Autodesk Inventor part; units mm, degrees
ref_plane "YZ Plane" through (0, 0, 0) normal (1, 0, 0) x (0, 1, 0)
ref_plane "XZ Plane" through (0, 0, 0) normal (0, 1, 0) x (-1, 0, 0)
ref_plane "XY Plane" through (0, 0, 0) normal (0, 0, 1) x (1, 0, 0)
sketch "Sketch1" plane through (0, 0, 0) normal (0, 1, 0) x (-1, 0, 0)
  line L0 (3.05, -5.3255) -> (-3.05, -5.3255)
  line L1 (-3.05, -5.3255) -> (-3.05, 4.8245)
  line L2 (-3.05, 4.8245) -> (3.05, 4.8245)
  line L3 (3.05, 4.8245) -> (3.05, -5.3255)
  line L4 (0.9, 4.8245) -> (-0.9, 4.8245)
  line L5 (0.9, 4.8245) -> (0.9, -5.3255)
  line L6 (-0.9, 4.8245) -> (-0.9, -5.3255)
  circle A0 centre (0, 3.486) radius 0.8
  circle A1 centre (-0.0087, -3.8255) radius 0.8
  line L7 (0, 4.8245) -> (0, -5.3255)
  line L8 (-3.05, 0) -> (3.05, 0)
  point P0 (0, 0)
  dimension "d13" = 6.1
  dimension "d44" = 1.8
  dimension "d45" = 2.15
  dimension "d46" = 1.6
  dimension "d47" = 1.6
extrude "Extrusion1" add sketch "Sketch1" along normal blind 10.15 contours L0 L5 L8 L3 | L0 L7 A1 L8 L5 | L8 L5 L2 L3 | L0 L6 L8 L7 A1 | L8 L7 A0 L2 L5 | L0 L1 L8 L6 | L8 L6 L2 L7 A0 | L8 L1 L2 L6
sketch "Sketch11" plane through (-3.05, 0, 4.8245) normal (0, 0, 1) x (1, 0, 0)
  point P0 (3.05, 0)
extrude "Extrusion6" add sketch "Sketch1" against normal blind 1 contours L0 L7 A1 L8 L5 | L0 L6 L8 L7 A1 | L8 L7 A0 L2 L5 | L8 L6 L2 L7 A0
sketch "Sketch12" plane through (0, 10.15, 0) normal (0, 1, 0) x (1, 0, 0)
  circle A0 centre (0.0087, 3.8255) radius 1.265
  circle A1 centre (0, -3.486) radius 1.265
  circle A2 centre (0, -3.486) radius 0.8
  circle A3 centre (0.0087, 3.8255) radius 0.8
  point P0 (0, 0)
  dimension "d52" = 2.53
  dimension "d53" = 2.53
extrude "Extrusion7" cut sketch "Sketch12" against normal blind 1 contours A0 | A1 | A2 | A3
sketch "Sketch13" plane through (-3.05, 10.15, 4.8245) normal (0, 0, 1) x (1, 0, 0)
  line L0 (0, 0) -> (0, -4.15)
  line L1 (0, -10.15) -> (0, 0)
  line L2 (0, -4.15) -> (6.1, -4.15)
  line L3 (6.1, -10.15) -> (6.1, 0)
  line L4 (6.1, 0) -> (6.1, -4.15)
  line L5 (0, 0) -> (6.1, 0)
  point P0 (3.05, -10.15)
  dimension "d56" = 4.15
extrude "Extrusion8" add sketch "Sketch13" along normal blind 17
sketch "Sketch17" plane through (-3.05, 10.15, 21.8245) normal (0, 0, 1) x (1, 0, 0)
  line L0 (6.1, 0) -> (0, 0)
  line L1 (6.1, 0) -> (14.3904, 5.5919)
  line L2 (6.1, 0) -> (16.1, 0) construction
  line L3 (14.3904, 5.5919) -> (10.1964, 11.8097)
  line L4 (10.1964, 11.8097) -> (13.5955, 14.1024)
  line L5 (13.5955, 14.1024) -> (17.7894, 7.8846)
  line L6 (17.7894, 7.8846) -> (19.7132, 5.0325)
  line L7 (6.1, -10.15) -> (6.1, -4.15)
  line L8 (19.7132, 5.0325) -> (6.1, -4.15)
  line L9 (6.1, 0) -> (6.1, -4.15)
  point P0 (3.05, -10.15)
  dimension "d72" = 10
  dimension "d73" = 34
  dimension "d74" = 7.5
  dimension "d75" = 4.1
extrude "Extrusion12" [suppressed]
sketch "Sketch14" plane through (0, 10.15, 0) normal (0, 1, 0) x (1, 0, 0)
  line L0 (3.05, 5.3255) -> (3.05, -21.8245)
  line L1 (3.05, -21.8245) -> (3.05, -17.7145)
  line L2 (3.05, -17.7145) -> (-3.05, -17.7145)
  line L3 (-3.05, 5.3255) -> (-3.05, -21.8245)
  line L4 (-3.05, -21.8245) -> (3.05, -21.8245)
  point P0 (0, 0)
  dimension "d59" = 4.11
extrude "Extrusion9" add sketch "Sketch14" along normal blind 9.25
sketch "Sketch16" plane through (0, 19.4, 0) normal (0, 1, 0) x (1, 0, 0)
  circle A0 centre (0, -19.7695) radius 1.5
  line L0 (-3.05, -21.8245) -> (3.05, -21.8245)
  line L1 (3.05, -21.8245) -> (3.05, -17.7145)
  point P0 (0, 0)
  point P1 (0, -21.8245)
  dimension "d67" = 3
  dimension "d68" = 2.055
  dimension "d69" = 3.05
extrude "Extrusion11" cut sketch "Sketch16" against normal blind 10
sketch "Sketch15" plane through (-3.05, 10.15, 21.8245) normal (0, 0, 1) x (1, 0, 0)
  line L0 (3.05, 7.25) -> (3.05, 4.45) construction
  line L1 (6.1, 0) -> (6.1, 9.25)
  line L2 (2.05, 7.25) -> (2.05, 4.45)
  line L3 (4.05, 4.45) -> (4.05, 7.25)
  arc A0 (4.05, 7.25) -> (2.05, 7.25) centre (3.05, 7.25) ccw
  arc A1 (2.05, 4.45) -> (4.05, 4.45) centre (3.05, 4.45) ccw
  line L4 (0, 9.25) -> (6.1, 9.25)
  line L5 (3.05, 9.25) -> (3.05, 8.25)
  point P0 (3.05, -10.15)
  point P1 (3.05, 5.85)
  dimension "d62" = 1.4
  dimension "d63" = 2
  dimension "d64" = 3.05
  dimension "d94" = 2.05
  dimension "d97" = 1
extrude "Extrusion10" cut sketch "Sketch15" against normal through all
sketch "Sketch20" plane through (10.5455, 24.2524, 21.8245) normal (-0.5591929, 0.8290376, 0) x (0.8290376, 0.5591929, 0)
  circle A0 centre (-2.05, 2.05) radius 1.5
  line L0 (-4.1, 0) -> (-4.1, 4.1)
  line L1 (0, 0) -> (-4.1, 0)
  point P0 (-22.3044, 21.8245)
  point P1 (-2.05, 0)
  dimension "d82" = 3
  dimension "d83" = 2.05
  dimension "d84" = 2.05
extrude "Extrusion14" [suppressed]
sketch "Sketch18" plane through (-3.05, 10.15, 21.8245) normal (0, 0, 1) x (1, 0, 0)
  line L0 (12.6984, 11.7664) -> (14.2641, 9.4451) construction
  line L1 (11.973, 11.2771) -> (13.5387, 8.9558)
  line L2 (14.9895, 9.9344) -> (13.4238, 12.2557)
  arc A0 (13.4238, 12.2557) -> (11.973, 11.2771) centre (12.6984, 11.7664) ccw
  arc A1 (13.5387, 8.9558) -> (14.9895, 9.9344) centre (14.2641, 9.4451) ccw
  line L3 (19.7132, 5.0325) -> (13.5955, 14.1024)
  line L4 (10.1964, 11.8097) -> (13.5955, 14.1024)
  point P0 (3.05, -10.15)
  point P1 (13.4813, 10.6057)
  point P2 (12.2091, 12.4918)
  dimension "d78" = 1.4
  dimension "d79" = 1.75
  dimension "d89" = 0.56
  dimension "d90" = 2.05
extrude "Extrusion13" cut sketch "Sketch18" against normal blind 4.1
sketch "Sketch21" plane through (13.8787, 15.6447, 19.7745) normal (-0.5591929, 0.8290376, 0) x (0.8290376, 0.5591929, 0)
  circle A0 centre (0, 0) radius 0.868
  point P0 (-20.2544, 19.7745)
extrude "Extrusion15" [suppressed]
mirror "Mirror3" about plane through (0, 0, 0) normal (1, 0, 0) of "Extrusion13"
fillet "Fillet1" radius 1 2 edges at (3.05, 10.15, 6.1945) (-3.05, 10.15, 6.1945)
fillet "Fillet2" [suppressed]
fillet "Fillet3" radius 1 2 edges at (3.05, 6, 13.3245) (-3.05, 6, 13.3245)
sketch "Sketch33" plane through (-3.05, 10.15, 21.8245) normal (0, 0, 1) x (1, 0, 0)
  line L0 (4.05, 7.25) -> (4.05, 4.45)
  arc A0 (2.05, 4.45) -> (4.05, 4.45) centre (3.05, 4.45) ccw
  line L1 (2.05, 4.45) -> (2.05, 7.25)
  arc A1 (4.05, 7.25) -> (2.05, 7.25) centre (3.05, 7.25) ccw
  arc A2 (0, -3.15) -> (1, -4.15) centre (1, -3.15) ccw
  line L2 (1, -4.15) -> (5.1, -4.15)
  arc A3 (5.1, -4.15) -> (6.1, -3.15) centre (5.1, -3.15) ccw
  line L3 (6.1, -3.15) -> (6.1, 9.25)
  line L4 (0, 9.25) -> (6.1, 9.25)
  line L5 (0, -3.15) -> (0, 9.25)
  point P0 (3.05, -10.15)
extrude "Extrusion17" add sketch "Sketch33" along normal blind 0.5
sketch "Sketch22" plane through (0, 9.4, 19.7695) normal (0, 1, 0) x (1, 0, 0)
  circle A0 centre (0, 0) radius 1.5
  point P0 (0, 19.7695)
extrude "Extrusion16" [suppressed]
equation "\"d13\" = base_width"
equation "\"d45\" = -0.5 * d44 + 0.5 * d13"
equation "\"d4\" = base_length"
equation "\"base_width\" = 6.1"
equation "\"base_length\" = 10.15"
equation "\"base_screw_diameter\" = 1.5"
equation "\"base_screw_spacing_edge\" = 8.5"
equation "\"multi_angle\" = 34deg"
properties part number "reinforced_holder"
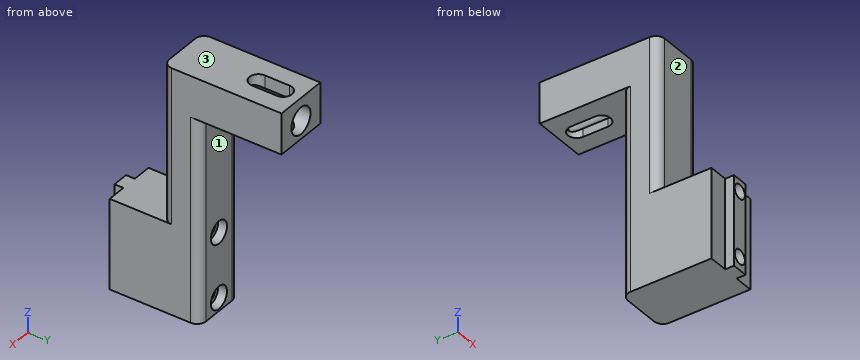
Here's how the part is built. I have some questions about the finished solid (model axes, mm). Face numbers are marked on the shaded views. A direction names the side the tool comes from. Coordinates: 2 decimals unless noted, no trailing zeros. Order: outer loops, then holes, each group sorted by start corner. A loop starts at its lowest first (then second) coordinate and runs counter-clockwise, first axis right, second up.
Item 1: If we section it at A-A, the plane y = 16.5: List the corners of the cut face in (x, z) for me.
Response values:
outline: (-3.05, 17.71) - (-1, 17.71) - (-1, 18.65) arc R1.5 cw to (-1, 20.89) - (-1, 22.32) - (-3.05, 22.32) - close; (1, 17.71) - (3.05, 17.71) - (3.05, 22.32) - (1, 22.32) - (1, 20.89) arc R1.5 cw to (1, 18.65) - close
Item 2: If we section it at D-D, the plane x = 2.5: List the corners of the cut face in (y, z) for me.
Response values:
outline: (0, -5.33) - (10.04, -5.33) - (10.04, 17.71) - (19.4, 17.71) - (19.4, 22.32) - (6.11, 22.32) - (6.11, 4.82) - (0, 4.82) - close
Item 3: I need wall thicknesses on probe 1 along Z at (x, y) = (0, 3.5); probe 2 along Y at (x, z) = (1.75, 7.25); probe 3 along X at (y, z) = (9, -3.75). Which ranges of each line are inside material? Lowest first, please.
Response values:
probe 1: z = -5.33 to -4.63, -3.03 to 2.69, 4.29 to 4.82
probe 2: y = 6 to 10.15
probe 3: x = -3.05 to -0.79, 0.81 to 3.05
Item 4: If we section it at C-C, the plane y = 11.25: List the corners of the cut face in (x, z) for me, then the cut area to 3 significant figures.
Response values:
outline: (-3.05, 17.71) - (3.05, 17.71) - (3.05, 22.32) - (-3.05, 22.32) - close; hole circle Ø3 at (0, 19.77)
area: 21.1 mm2
Item 5: If we section it at B-B, the plane z = 8: List the corners of the cut face in (x, y) for me, then the cut area to 3 significant figures.
Response values:
outline: (-3.05, 7) arc R1 ccw to (-2.05, 6) - (2.05, 6) arc R1 ccw to (3.05, 7) - (3.05, 9.15) arc R1 ccw to (2.05, 10.15) - (-2.05, 10.15) arc R1 ccw to (-3.05, 9.15) - close
area: 24.5 mm2
Item 6: I'm going to push flat-ended pins straight in: pin 1 Ø1.5 at (x, z) = (0.01, -3.83) entering from +Y; pin 2 Ø1.1 at (x, z) = (-1.5, 1.5) entering from -Y; pin 3 Ø3.5 at (x, z) = (0.5, 8.5) entering from +Y; pin 4 Ø3.5 at (x, z) = (-0.5, 16.5) entering from -Y. Where does each tip first touch, or does it pass through?
Response values:
pin 1: passes through
pin 2: stops at y = 0
pin 3: stops at y = 10.15
pin 4: stops at y = 6
Item 7: Which directions (+Z, -Z, +X, -X, +Y, -Y) give clear straight access to the entire face, cutting with the end or side of a thin tool? Please do the marked faces 1, 2 and 3.
Response values:
face 1: -Z, +X, -X, +Y
face 2: +Z, +X, -X, -Y
face 3: +Z, +X, -X, +Y, -Y
